from build123d import *

# Parameters (mm, degrees)
BOSS_EXTRUDE1_DEPTH              = 9.525
SKETCH2_R                        = 3.302
CUT_EXTRUDE1_DEPTH               = 19.05
F_25_64_0_39063_DIAMETER_HOLE1_D = 9.922002


with BuildPart() as part:
    # Sketch1 → Boss-Extrude1 (new body, symmetric)
    with BuildSketch(Plane.XY):
        with BuildLine():
            Line((-80.658868274, 131.257470336), (-31.489028268, 201.479279332))
            ThreePointArc((-31.489028268, 201.479279332), (-66.529224029, 183.480200423), (-100.606355042, 163.718335568))
            ThreePointArc((-100.606355042, 163.718335568), (-175.90250014, 77.354007785), (-188.658870504, -36.5125))
            Line((-188.658870504, -36.5125), (-149.670350751, -36.5125))
            ThreePointArc((-149.670350751, -36.5125), (-142.476587623, 58.607154251), (-80.658868274, 131.257470336))
        make_face()
    extrude(amount=BOSS_EXTRUDE1_DEPTH, both=True)

    # Sketch2 → Cut-Extrude1 (cut)
    with BuildSketch(Plane.XY.offset(9.525)):
        with Locations((-173.718655592, 7.579557452)):
            Circle(SKETCH2_R)
        with Locations((-166.564839951, 51.569288407)):
            Circle(SKETCH2_R)
    extrude(amount=-CUT_EXTRUDE1_DEPTH, mode=Mode.SUBTRACT)

    # 25/64 (0.39063) Diameter Hole1 (through all)
    with Locations(Plane.XY.offset(9.525)):
        with Locations((-103.331077236, 129.637230364), (-157.212613963, 75.755693637)):
            Hole(F_25_64_0_39063_DIAMETER_HOLE1_D / 2)


solid = part.part
Verification items for the finished model (mm, model axes). Coordinates: 2 decimals unless noted, no trailing zeros. Write each loop counter-clockwise with the first axis right and the second up, starting at its lowest first coordinate (ties: lowest second). Pieces come first, ordered by that corner, then holes. Notation, with made-up numbers: (-0.75, 24.5) -> (32.25, 24.5) arc R13 ccw to (32.25, 30.5) -> close; hole circle Ø7 at (11.25, -22). An arc over 180 degrees is marked (long way). One line per item, written item: value. Start each with the question number.
Q1. Cross-section at C-C on x = -140. Enter the section's corners in (y, z) (3 decimals).
Q2. Mould release check, pull along X, two halves, no side actions. Record for faces 1 (the flat face through (-56.4, 165.9, 0.1)), 2 (the cylindrical face through (-152.256, 75.974, -0.133)), 3 (the flat face through (-169, -36.512, 0)), 4 (the cylindrical face through (-175.24, 78.84, 0.13)): pulls with the +X half, pulls with the -X half, needs draft (parallel to the pull), parting line crosses it, or undercut.
Q3. Cross-section at B-B on y = -8. Enter the section's corners in (x, z) (3 decimals), and give its area (3 significant figures).
Q4. Cross-section at A-A on z = 0. Enter the section's corners in (x, y), and give its area (3 significant figures).
Q5. Go/stop test with flat-tipped pins: P1, Ø1, axis at y = -9.5, z = 6, coming from the -X side; P2, Ø1.5, axis at y = 53.5, z = 3.5, coming from the -X side; P3, Ø2, axis at y = 105, z = -6, coming from the +X side. Record where each tip stops, or that it passes through.
Q6. Thickness scan on L1, parallel to Y at x = -107, z = -0.25; L2, parallel to X at y = 50.5, z = -3.75; L3, parallel to Y at x = -172, z = -8. Record the ranges inside material, lowest first. Write a range as from..to.
Checked values:
1. outline: (64.299, -9.525) -> (131.626, -9.525) -> (131.626, 9.525) -> (64.299, 9.525) -> close
2. face 1: pulls with the +X half
2. face 2: undercut
2. face 3: needs draft
2. face 4: pulls with the -X half
3. outline: (-191.993, -9.525) -> (-153.852, -9.525) -> (-153.852, 9.525) -> (-191.993, 9.525) -> close
3. area: 727 mm²
4. outline: (-188.66, -36.51) -> (-149.67, -36.51) arc R154.06 cw to (-80.66, 131.26) -> (-31.49, 201.48) arc R772.53 ccw to (-100.61, 163.72) arc R192.16 ccw to start; hole circle Ø6.6 at (-173.72, 7.58); hole circle Ø6.6 at (-166.56, 51.57); hole circle Ø9.92 at (-157.21, 75.76); hole circle Ø9.92 at (-103.33, 129.64)
4. area: 9,460 mm²
5. P1: stops at x = -191.95
5. P2: stops at x = -184.78
5. P3: stops at x = -111.8
6. L1: y = 110.84..126.3, 132.98..159.61
6. L2: x = -185.41..-169.69, -163.44..-145.55
6. L3: y = -36.51..4.76, 10.4..85.68
